from build123d import *

# Parameters (mm, degrees)
SKIZZE1_R                            = 5
ZYLINDER_DEPTH                       = 2.2
SCHNITT_LINEAR_AUSTRAGEN1_DEPTH      = 10
SCHNITT_LINEAR_AUSTRAGEN1_DEPTH_BACK = 5
SKIZZE4_R                            = 4.5
SKIZZE6_R                            = 22.5
FASSUNG_OBJEKTTR_GERGEWINDE_DEPTH    = 7
SKIZZE11_R                           = 20.3
BOHRUNG_F_R_INNENGEWINDE_DEPTH       = 6
SKIZZE13_R                           = 6
AUFSATZ_LINEAR_AUSTRAGEN1_DEPTH      = 3
SKIZZE16_R                           = 2.6
SCHNITT_LINEAR_AUSTRAGEN13_DEPTH     = 10
GEWINDE1_PITCH                       = 1.5
SKIZZE17_W                           = 26.5
SKIZZE17_H                           = 49.541135346
SCHNITT_LINEAR_AUSTRAGEN14_DEPTH     = 1.6


with BuildPart() as part:
    # Skizze1 → Zylinder (new body)
    with BuildSketch(Plane(origin=(0, 0, 0), x_dir=(1, 0, 0), z_dir=(0, 1, 0))):
        with Locations(Location((-18.043745097, 0, 0), (0, 0, 270))):
            Circle(SKIZZE1_R)
    extrude(amount=ZYLINDER_DEPTH)

    # Skizze4 → Schnitt-Linear austragen1 (cut, two sides: drawn at the far end of the back side and taken through both)
    with BuildSketch(Plane(origin=(0, 2.2, 0), x_dir=(1, 0, 0), z_dir=(0, 1, 0)).offset(-SCHNITT_LINEAR_AUSTRAGEN1_DEPTH_BACK)):
        with Locations(Location((-18.043745097, 0, 0), (0, 0, 270))):
            Circle(SKIZZE4_R)
    extrude(amount=SCHNITT_LINEAR_AUSTRAGEN1_DEPTH + SCHNITT_LINEAR_AUSTRAGEN1_DEPTH_BACK, mode=Mode.SUBTRACT)

    # Skizze6 → Fassung Objektträgergewinde (add)
    with BuildSketch(Plane(origin=(0, 0, 0), x_dir=(-1, 0, 0), z_dir=(0, -1, 0))):
        with Locations(Location((18.043745097, 0, 0), (0, 0, 90))):
            Circle(SKIZZE6_R)
    extrude(amount=FASSUNG_OBJEKTTR_GERGEWINDE_DEPTH)

    # Skizze11 → Bohrung für Innengewinde (cut)
    with BuildSketch(Plane(origin=(0, -7, 0), x_dir=(-1, 0, 0), z_dir=(0, -1, 0))):
        with Locations(Location((18.043745097, 0, 0), (0, 0, 90))):
            Circle(SKIZZE11_R)
    extrude(amount=-BOHRUNG_F_R_INNENGEWINDE_DEPTH, mode=Mode.SUBTRACT)

    # Skizze13 → Aufsatz-Linear austragen1 (add)
    with BuildSketch(Plane(origin=(0, 0, 0), x_dir=(-1, 0, 0), z_dir=(0, -1, 0))):
        with Locations(Location((18.043745097, 0, 0), (0, 0, 90))):
            Circle(SKIZZE13_R)
    extrude(amount=-AUFSATZ_LINEAR_AUSTRAGEN1_DEPTH)

    # Skizze16 → Schnitt-Linear austragen13 (cut)
    with BuildSketch(Plane(origin=(0, -7, 0), x_dir=(-1, 0, 0), z_dir=(0, -1, 0))):
        with Locations(Location((18.043745097, 0, 0), (0, 0, 90))):
            Circle(SKIZZE16_R)
    extrude(amount=-SCHNITT_LINEAR_AUSTRAGEN13_DEPTH, mode=Mode.SUBTRACT)

    # Gewinde1: the profile of Gewindeprofil1 profile screwed along a right-hand helix of 2.333333 turns, 8 arcs to a turn; built about Z, then put on its axis
    gewinde1_z = Axis((0, 0, 0), (0, 0, 1))
    gewinde1_corners = [(6.0003, 0, -0.000173205), (6.0003, 0, 1.312673201), (5.188101187, 0, 0.843749998), (5.188101187, 0, 0.468749998)]
    with BuildLine(mode=Mode.PRIVATE) as gewinde1_profile:
        Line(gewinde1_corners[0], gewinde1_corners[1])
        Line(gewinde1_corners[1], gewinde1_corners[2])
        Line(gewinde1_corners[2], gewinde1_corners[3])
        Line(gewinde1_corners[3], gewinde1_corners[0])
    gewinde1_cap = Face(gewinde1_profile.wire())
    gewinde1_turn_angles = [0, 22.5, 45, 67.5, 90, 112.5, 135, 157.5, 180, 202.5, 225, 247.5, 270, 292.5, 315, 337.5, 360]
    gewinde1_turn_weights = [1, 0.9238795325112867, 1, 0.9238795325112867, 1, 0.9238795325112867, 1, 0.9238795325112867, 1, 0.9238795325112867, 1, 0.9238795325112867, 1, 0.9238795325112867, 1, 0.9238795325112867, 1]
    gewinde1_turn_rails = [Edge.make_bspline([Vector(p[0], p[1], 0).rotate(gewinde1_z, gewinde1_turn_angles[k]) / gewinde1_turn_weights[k] + Vector(0, 0, p[2] + GEWINDE1_PITCH * gewinde1_turn_angles[k] / 360) for k in range(17)], [0, 0, 0, 1, 1, 2, 2, 3, 3, 4, 4, 5, 5, 6, 6, 7, 7, 8, 8, 8], 2, gewinde1_turn_weights) for p in gewinde1_corners]
    gewinde1_turn_sides = [Face.make_surface_from_curves(gewinde1_turn_rails[p[0]], gewinde1_turn_rails[p[1]]) for p in [(0, 1), (1, 2), (2, 3), (3, 0)]]
    gewinde1_last_angles = [720, 742.5, 765, 787.5, 810, 825, 840]
    gewinde1_last_weights = [1, 0.9238795325112867, 1, 0.9238795325112867, 1, 0.9659258262890685, 1]
    gewinde1_last_rails = [Edge.make_bspline([Vector(p[0], p[1], 0).rotate(gewinde1_z, gewinde1_last_angles[k]) / gewinde1_last_weights[k] + Vector(0, 0, p[2] + GEWINDE1_PITCH * gewinde1_last_angles[k] / 360) for k in range(7)], [0, 0, 0, 1, 1, 2, 2, 3, 3, 3], 2, gewinde1_last_weights) for p in gewinde1_corners]
    gewinde1_last_sides = [Face.make_surface_from_curves(gewinde1_last_rails[p[0]], gewinde1_last_rails[p[1]]) for p in [(0, 1), (1, 2), (2, 3), (3, 0)]]
    gewinde1 = Plane(origin=(-18.043745097, 4.6, 0), x_dir=(-1, 0, 0), z_dir=(0, -1, 0)) * Solid(Shell([*[p.moved(Location((0, 0, GEWINDE1_PITCH * i))) for i in range(2) for p in gewinde1_turn_sides], *gewinde1_last_sides, gewinde1_cap, gewinde1_cap.rotate(gewinde1_z, 840).moved(Location((0, 0, GEWINDE1_PITCH * 840 / 360)))]))
    add(gewinde1, mode=Mode.SUBTRACT)

    # Skizze17 → Schnitt-Linear austragen14 (cut)
    with BuildSketch(Plane(origin=(0, -2, 0), x_dir=(1, 0, 0), z_dir=(0, 1, 0))):
        with Locations((-18.043745097, 0)):
            Rectangle(SKIZZE17_W, SKIZZE17_H)
    extrude(amount=-SCHNITT_LINEAR_AUSTRAGEN14_DEPTH, mode=Mode.SUBTRACT)


solid = part.part
The listing builds one solid part. Answer for the finished solid, in the listing's coordinates (mm). A direction names the side the tool comes from. Coordinates: 2 decimals unless noted, no trailing zeros. Write each loop counter-clockwise with the first axis right and the second up, starting at its lowest first coordinate (ties: lowest second). Pieces come first, ordered by that corner, then holes. Notation, with made-up numbers: M -12,-34 L 13,-34 A5 ccw 13,-27 Z; hole C -4.5,44.5 d4. An arc over 180 degrees is marked long. Use one line per item in the form item = value.
Item 1: Given P1, Ø2, axis at x = -23.5, z = -19.5, coming from the +Y side; P2, Ø20.5, axis at x = -17, z = 9.5, coming from the -Y side; P3, Ø1.8, axis at y = -2.5, z = 16.5, coming from the +X side; P4, Ø5, axis at x = -16, y = -4, coming from the +Z side, each flat-ended and moving along its own axis, determine where each tip first touches the part or whether it passes through.
Model answer:
P1 = 0
P2 = -1
P3 = -1.83
P4 = 22.5
Item 2: Find section A-A, the plane x = -28. Give the vertices of the cut face in (y, z), plus the area to 3 significant figures.
Model answer:
outline = M -7,-20.18 L -3.6,-20.18 L -3.6,-17.69 L -7,-17.69 Z; M -7,17.69 L -3.6,17.69 L -3.6,20.18 L -7,20.18 Z; M -2,-20.18 L 0,-20.18 L 0,20.18 L -2,20.18 L -2,17.69 L -1,17.69 L -1,-17.69 L -2,-17.69 Z
area = 62.2 mm2
Item 3: Find section D-D, the plane x = -11.5. Give the vertices of the cut face in (y, z), plus the area to 3 significant figures.
Model answer:
outline = M -7,-21.53 L -3.6,-21.53 L -3.6,-19.22 L -7,-19.22 Z; M -7,19.22 L -3.6,19.22 L -3.6,21.53 L -7,21.53 Z; M -2,-21.53 L 0,-21.53 L 0,21.53 L -2,21.53 L -2,19.22 L -1,19.22 L -1,-19.22 L -2,-19.22 Z
area = 63.4 mm2
Item 4: Find section C-C, the plane z = 16.5. Give the vertices of the cut face in (x, y), plus the area to 3 significant figures.
Model answer:
outline = M -33.34,-7 L -29.87,-7 L -29.87,-3.6 L -31.29,-3.6 L -31.29,-2 L -29.87,-2 L -29.87,-1 L -6.22,-1 L -6.22,-2 L -4.79,-2 L -4.79,-3.6 L -6.22,-3.6 L -6.22,-7 L -2.75,-7 L -2.75,0 L -33.34,0 Z
area = 67.7 mm2
Item 5: Find section B-B, the plane y = -6. Give the vertices of the cut face in (x, z).
Model answer:
outline = C -18.04,0 d45; hole C -18.04,0 d40.6
Item 6: Find the intervals of material crossed by probe 1 along X at (y, z) = (-5.05, 0); probe 2 along Y at (x, z) = (-26.5, -14.5); probe 3 along Z at (x, y) = (-28, -4.5), in increasing order.
Model answer:
probe_1 = -40.54 to -38.34, 2.26 to 4.46
probe_2 = -1 to 0
probe_3 = -20.18 to -17.69, 17.69 to 20.18
Item 7: For faces 4 (the face through (-21, 3, 0)), 5 (the face through (-17, -2, -21)), 6 (the face through (-22, -1, 0)), determine the directions among +Z, -Z, +X, -X, +Y, -Y from which every point of the face is accessible in a straight line to the end or side of a thin tool.
Model answer:
face_4 = +Z, -Z, +X, -X, +Y
face_5 = +Z, -Z
face_6 = -Y
Item 8: The mould has two halves that part along Z. Classify faces 1 (the face through (-23, 0, -5)), 2 (the face through (2.084, -4.042, 2.643)), 3 (the face through (-17.05, -4.23, 22.48)): released by +Z, released by -Z, zero draft, split by the parting line, or undercut.
Model answer:
face_1 = zero draft
face_2 = undercut
face_3 = split by the parting line
